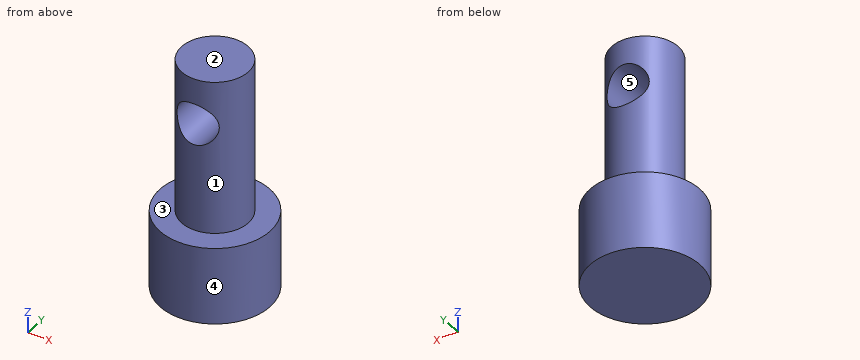
from build123d import *

# Parameters (mm, degrees)
F0_R          = 3.55
F1_DEPTH      = 5
F2_R          = 2.15
F3_DEPTH      = 10
F4_R          = 1.35
F5_DEPTH      = 2.15
F5_DEPTH_BACK = 2.15


with BuildPart() as f1:
    # F0 (on Top) → F1 (new body)
    with BuildSketch(Plane.XY):
        Circle(F0_R)
    extrude(amount=F1_DEPTH)

    # F2 (on face) → F3 (join)
    with BuildSketch(Plane.XY.offset(5)):
        Circle(F2_R)
    extrude(amount=F3_DEPTH)

    # F4 (on Front) → F5 (cut, two sides)
    with BuildSketch(Plane.XZ) as f5_sk:
        with Locations((0, 12)):
            Circle(F4_R)
    extrude(amount=-F5_DEPTH, mode=Mode.SUBTRACT)
    extrude(f5_sk.sketch, amount=F5_DEPTH_BACK, mode=Mode.SUBTRACT)


solid = f1.part
Part model, mm, in its own coordinate system. Face numbers are marked on the shaded views. A direction names the side the tool comes from. Coordinates: 2 decimals unless noted, no trailing zeros. Order: outer loops, then holes, each group sorted by start corner. A loop starts at its lowest first (then second) coordinate and runs counter-clockwise, first axis right, second up. Notation, with made-up numbers: M 68.5,-6.75 L 74.5,-6.75 A9 ccw 74.5,7.25 Z; hole C 36.5,5.25 d9. An arc over 180 degrees is marked long. Use a Markdown table: item, result.
(1) Probe L1, parallel to Z at x = 0, y = -1; L2, parallel to X at y = 0.55, z = 12; L3, parallel to X at y = 0.85, z = 12. List the from-to ranges inside material, lowest first.
A:
| item | result |
|---|---|
| L1 | z = 0 to 10.65, 13.35 to 15 |
| L2 | x = -2.08 to -1.35, 1.35 to 2.08 |
| L3 | x = -1.97 to -1.35, 1.35 to 1.97 |
(2) Tool access for the marked faces 1 and 2: list every direction of +Z, -Z, +X, -X, +Y, -Y with a clear straight run to the whole face (end or side of a thin tool).
A:
| item | result |
|---|---|
| face 1 | +Z |
| face 2 | +Z, +X, -X, +Y, -Y |
(3) Cut at D-D on x = 0.75. Write the cut outline in (y, z).
A:
| item | result |
|---|---|
| outline | M -3.47,0 L 3.47,0 L 3.47,5 L 2.01,5 L 2.01,10.88 L -2.01,10.88 L -2.01,5 L -3.47,5 Z; M -2.01,13.12 L 2.01,13.12 L 2.01,15 L -2.01,15 Z |
(4) Cut at A-A on x = 0. Write the cut outline in (y, z).
A:
| item | result |
|---|---|
| outline | M -3.55,0 L 3.55,0 L 3.55,5 L 2.15,5 L 2.15,10.65 L -2.15,10.65 L -2.15,5 L -3.55,5 Z; M -2.15,13.35 L 2.15,13.35 L 2.15,15 L -2.15,15 Z |
(5) Cut at C-C on z = 12. Write the cut outline in (x, y).
A:
| item | result |
|---|---|
| outline | M -1.35,-1.67 L -1.35,1.67 A2.15 ccw Z; M 1.35,-1.67 A2.15 ccw 1.35,1.67 Z |
(6) Flat gauge pins, fed straight in: pin 1 (1.5 mm diameter, centred on x = -2, z = 3, fed in from +Y); pin 2 (3.5 mm diameter, centred on x = 0, z = 12, fed in from -Y); pin 3 (1.5 mm diameter, centred on x = 2, z = 5.5, fed in from +Y). Where does each tip first touch, or does it go through?
A:
| item | result |
|---|---|
| pin 1 | stops at y = 3.32 |
| pin 2 | stops at y = -2.15 |
| pin 3 | stops at y = 3.24 |
(7) Pull direction X, two halves, no side cores. Call the marked faces 3, 4 and 5: released by +X, released by -X, zero draft, split by the parting line, or undercut.
A:
| item | result |
|---|---|
| face 3 | zero draft |
| face 4 | split by the parting line |
| face 5 | undercut |
(8) Cut at B-B on y = 0. Write the cut outline in (x, z).
A:
| item | result |
|---|---|
| outline | M -3.55,0 L 3.55,0 L 3.55,5 L 2.15,5 L 2.15,15 L -2.15,15 L -2.15,5 L -3.55,5 Z; hole C 0,12 d2.7 |
